Work out the finished part from the listing and answer in its coordinate system (mm). Round coordinates to 2 decimals unless told otherwise and drop trailing zeros. Order: outer loops, then holes, each group sorted by start corner. A loop starts at its lowest first (then second) coordinate and runs counter-clockwise, first axis right, second up. Notation, with made-up numbers: (61, 58) - (102, 58) arc R19 cw to (102, 92) - close; hole circle Ø3 at (-31, 77.25). An arc over 180 degrees is marked (long way). One line per question, with ' | ' between items. Start each with the question number.
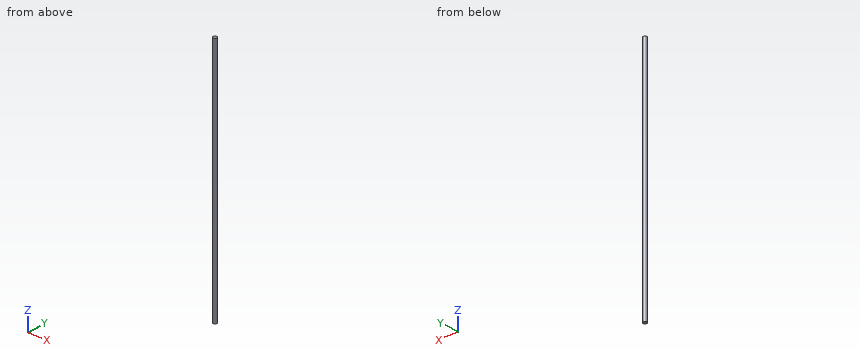
from build123d import *

# Parameters (mm, degrees)
SKETCH1_R                    = 6.35
BOSS_EXTRUDE1_DEPTH          = 914.4
ENL_V_START                  = -34.29
ESQUISSE1_R                  = 6.35
ENL_V_MAT_EXTRU_1_DEPTH      = 34.29
ENL_V_MAT_EXTRU_3_DEPTH      = 881.155814103
ENL_V_MAT_EXTRU_3_DEPTH_BACK = 881.155814103
ESQUISSE3_W                  = 12.7
ESQUISSE3_H                  = 38.1


with BuildPart() as part:
    # Sketch1 → Boss-Extrude1 (new body)
    with BuildSketch(Plane.XY):
        Circle(SKETCH1_R)
    extrude(amount=BOSS_EXTRUDE1_DEPTH)

    # Esquisse1 → Enlèv. mat.-Extru.1 (cut)
    with BuildSketch(Plane.XY.offset(914.4).offset(ENL_V_START)):
        Circle(ESQUISSE1_R)
    extrude(amount=ENL_V_MAT_EXTRU_1_DEPTH, mode=Mode.SUBTRACT)

    # Esquisse3 → Enlèv. mat.-Extru.3 (cut, two sides: drawn at the far end of the back side and taken through both)
    with BuildSketch(Plane(origin=(0, 0, 0), x_dir=(1, 0, 0), z_dir=(0, 1, 0)).offset(-ENL_V_MAT_EXTRU_3_DEPTH_BACK)):
        with Locations((0, -19.05)):
            Rectangle(ESQUISSE3_W, ESQUISSE3_H)
    extrude(amount=ENL_V_MAT_EXTRU_3_DEPTH + ENL_V_MAT_EXTRU_3_DEPTH_BACK, mode=Mode.SUBTRACT)


solid = part.part
1) Flat-ended cylindrical pins translate along their axes: pin 1 (3 mm diameter, centred on y = -0.5, z = 433, fed in from +X); pin 2 (4 mm diameter, centred on x = -3, z = 646.5, fed in from +Y); pin 3 (1.5 mm diameter, centred on x = 1, z = 712.5, fed in from -Y). Find the tip coordinate at first contact, or state that the pin passes through.
2) Section A-A on z = 501.5 is taken. Give the vertices of the cut face in (x, y).
3) Straight lines are drawn through the part: line 1 (X direction, y = 0.5, z = 201.5); line 2 (X direction, y = 1.25, z = 159). For each, find the intervals that lie inside material, in ascending order.
4) Section B-B on x = 2 is taken. Give the vertices of the cut face in (y, z), and give its area (3 significant figures).
Recorded:
1) pin 1: stops at x = 6.35 | pin 2: stops at y = 6.27 | pin 3: stops at y = -6.35
2) outline: circle Ø12.7 at (0, 0)
3) line 1: x = -6.33 to 6.33 | line 2: x = -6.23 to 6.23
4) outline: (-6.03, 38.1) - (6.03, 38.1) - (6.03, 880.11) - (-6.03, 880.11) - close | area: 10,100 mm²
